Autodesk Inventor part; units mm, degrees
ref_plane "YZ Plane" through (0, 0, 0) normal (1, 0, 0) x (0, 1, 0)
ref_plane "XZ Plane" through (0, 0, 0) normal (0, 1, 0) x (-1, 0, 0)
ref_plane "XY Plane" through (0, 0, 0) normal (0, 0, 1) x (1, 0, 0)
sketch "Boceto1" plane through (0, 0, 0) normal (1, 0, 0) x (0, 1, 0)
  line L0 (0, 0) -> (-525, 0)
  line L1 (-525, 0) -> (-525, -6.4)
  line L2 (-525, -6.4) -> (0, -6.4)
  line L3 (0, -6.4) -> (0, 0)
  line L4 (-525, -6.4) -> (-354, -6.4)
  line L5 (-354, -6.4) -> (-354, -7.7448)
  line L6 (-354, -6.4) -> (-354, -437.06)
  line L7 (-354, -6.4) -> (-360.4, -6.4)
  line L8 (-360.4, -6.4) -> (-360.4, -437.06)
  line L9 (0, -443.46) -> (-525, -443.46)
  line L10 (-525, -443.46) -> (-525, -437.06)
  line L11 (-525, -437.06) -> (0, -437.06)
  line L12 (0, -437.06) -> (0, -443.46)
  line L13 (-354, -437.06) -> (-74, -437.06)
  line L14 (-74, -437.06) -> (-74, -6.4)
  line L15 (-74, -437.06) -> (-67.6, -437.06)
  line L16 (-67.6, -437.06) -> (-67.6, -6.4)
  dimension "d0" = 525
  dimension "d1" = 6.4
  dimension "d2" = 171
  dimension "d3" = 430.66
  dimension "d4" = 6.4
  dimension "d5" = 430.66
  dimension "d6" = 280
  dimension "d7" = 6.4
extrude "Extrusión1" add sketch "Boceto1" along normal blind 25.4 contours L3 L2 L1 L0 | L16 L11 L14 L2 | L2 L5 L6 L11 L8 | L11 L12 L9 L10
sketch "Boceto2" plane through (0, -525, 0) normal (0, 0, 1) x (1, 0, 0)
  line L0 (0, 525) -> (0, 523.23)
  line L1 (0, 525) -> (0, 0)
  line L2 (0, 523.23) -> (25.4, 523.23)
  line L3 (25.4, 525) -> (25.4, 0)
  line L4 (25.4, 525) -> (0, 525)
  dimension "d10" = 1.77
extrude "Extrusión2" cut sketch "Boceto2" against normal through all
sketch "Boceto3" plane through (0, -525, 0) normal (0, 0, 1) x (1, 0, 0)
  line L0 (0, 523.23) -> (25.4, 523.23)
  line L1 (25.4, 523.23) -> (25.4, 514.5)
  line L2 (25.4, 0) -> (25.4, 523.23)
  line L3 (25.4, 514.5) -> (12.7, 514.5)
  circle A0 centre (12.7, 514.5) radius 1
  point P0 (0, 525)
  dimension "d13" = 8.73
  dimension "d14" = 12.7
  dimension "d15" = 2
extrude "Extrusión3" cut sketch "Boceto3" against normal through all
properties part number "Soporte_molde"
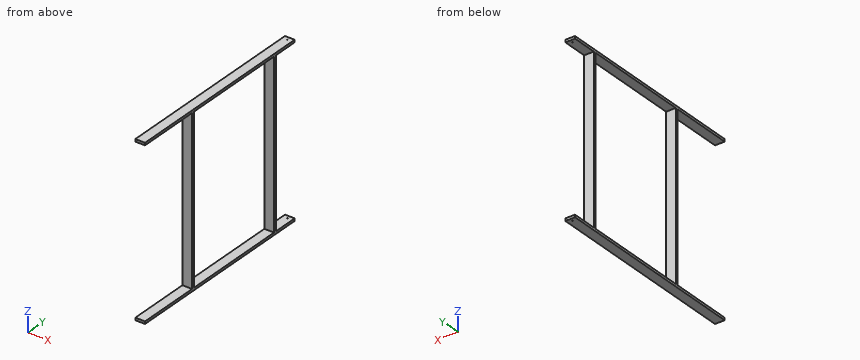
Model file for the job. Use its own axes, mm. Give positions to 0.01 mm unless a question says otherwise; leave off trailing zeros. Loops run counter-clockwise (first coordinate to the right, second up) from the corner with the lowest first, then second, coordinate; pieces in that order, holes last. Notation, with made-up numbers: (6, -7) - (37, -7) arc R23 cw to (37, 19) - close; hole circle Ø10 at (-34, 39.5). An arc over 180 degrees is marked (long way). Use one line per item in the form item = value.
(1) Drill centre lines: L1, parallel to Y at x = 12.7, z = -2; L2, parallel to Y at x = 20.5, z = -363; L3, parallel to Z at x = 1.5, y = -64.5. Where is each one in solid material? Low to high.
Determined:
L1 = -525 to -11.5, -9.5 to -1.77
L2 = -360.4 to -354, -74 to -67.6
L3 = -443.46 to -437.06, -6.4 to 0
(2) Cut at B-B (y = -379). Give the cut face in (x, z), then the cut area to 3 significant figures.
Determined:
outline = (0, -443.46) - (25.4, -443.46) - (25.4, -437.06) - (0, -437.06) - close; (0, -6.4) - (25.4, -6.4) - (25.4, 0) - (0, 0) - close
area = 325 mm^2
(3) Drop flat-ended pins along their axis: P1, Ø12.5, axis at x = 10, z = -122, coming from the +Y side; P2, Ø1, axis at x = 18.5, z = -367.5, coming from the -Y side. Give the stop position or say it passes through.
Determined:
P1 = -67.6
P2 = -360.4
(4) Cut at A-A (z = -216). Give the cut face in (x, y).
Determined:
outline = (0, -360.4) - (25.4, -360.4) - (25.4, -354) - (0, -354) - close; (0, -74) - (25.4, -74) - (25.4, -67.6) - (0, -67.6) - close
(5) Cut at C-C (x = 19.5). Give the cut face in (y, z), then the cut area to 3 significant figures.
Determined:
outline = (-525, -443.46) - (-1.77, -443.46) - (-1.77, -437.06) - (-67.6, -437.06) - (-67.6, -6.4) - (-1.77, -6.4) - (-1.77, 0) - (-525, 0) - (-525, -6.4) - (-360.4, -6.4) - (-360.4, -437.06) - (-525, -437.06) - close; hole (-354, -437.06) - (-74, -437.06) - (-74, -6.4) - (-354, -6.4) - close
area = 12,200 mm^2
